Here's how the part is built. I have some questions about the finished solid (model axes, mm). A direction names the side the tool comes from. Coordinates: 2 decimals unless noted, no trailing zeros. Loops run counter-clockwise (first coordinate to the right, second up) from the corner with the lowest first, then second, coordinate; pieces in that order, holes last. Notation, with made-up numbers: M 52.5,42.5 L 66.5,42.5 A8 cw 66.5,53.5 Z; hole C 13.5,-8.75 d1. An arc over 180 degrees is marked long. Use one line per item in the form item = value. Start each with the question number.
(1) Imagine slicing it at C-C, the plane y = 15. Please give me the cut outline in (x, z).
(2) Imagine slicing it at A-A, the plane x = 0. Please give me the cut outline in (y, z) (3 decimals), and give its area (3 significant figures).
(3) Imagine slicing it at B-B, the plane z = 0. Please give me the cut outline in (x, y).
(4) On a 3-axis mill with a long thin cutter (end or side, diameter ignored), from which of +Z, -Z, +X, -X, +Y, -Y can I reach the whole of each face in a straight line? I mean faces 5 (the flat face through (-10.795, 6, -37)), 6 (the flat face through (26.87, 6.44, 27.98)), 7 (the cylindrical face through (-1.686, 5.106, -31.791)). Say none if no direction works.
(5) Imagine slicing it at D-D, the plane z = -16. Please give me the cut outline in (x, y), and give its area (3 significant figures).
(6) Thinking about a two-plate mould opening in Y: for faces 1 (the cylindrical face through (-0.237, 23.492, -37.256)), 2 (the flat face through (-37.7, 6.4, 9.3)), 3 (the cylindrical face through (25.737, 5.799, 19.004)), 4 (the cylindrical face through (-26.689, 5.106, 17.356)), which applies, +Y half, -Y half, draft (parallel to the pull), parting line (faces both ways), or undercut?
(7) Will these pins go through, and if not, where does the flat tip stop? P1, Ø12, axis at x = 32, z = -28, coming from the +Y side (1 decimal); P2, Ø2, axis at y = 45.5, z = -3, coming from the -X side; P3, Ø12, axis at y = 35.5, z = -22, coming from the +X side; P4, Ø5, axis at x = 9.5, z = -33.5, coming from the +Y side.
(8) Please list where these lines run through material, in increasing order: L1, parallel to X at y = 12.7, z = -37.5 (3 decimals); L2, parallel to X at y = 20.5, z = 2; L3, parallel to X at y = 7, z = 16.5.
```python
from build123d import *

# Parameters (mm, degrees)
SKETCH1_R               = 31.75
SKETCH1_R_2             = 20.32
BOSS_EXTRUDE1_DEPTH     = 50.8
BOSS_EXTRUDE2_START     = -12.7
SKETCH2_R               = 7.77875
BOSS_EXTRUDE2_DEPTH     = 14.591493
SKETCH2_2_R             = 7.77875
CUT_EXTRUDE1_DEPTH      = 12.977852
CIRPATTERN1_COUNT       = 3
F_1_4_CLEARANCE_HOLE1_D = 7.14248


with BuildPart() as part:
    # Sketch1 → Boss-Extrude1 (new body)
    with BuildSketch(Plane(origin=(0, 0, 0), x_dir=(1, 0, 0), z_dir=(0, 1, 0))):
        Circle(SKETCH1_R)
        Circle(SKETCH1_R_2, mode=Mode.SUBTRACT)
    extrude(amount=BOSS_EXTRUDE1_DEPTH)

    # Sketch2 → Boss-Extrude2 (add)
    with BuildSketch(Plane.XY.offset(-31.75).offset(BOSS_EXTRUDE2_START)):
        with BuildLine():
            Line((10.795, 12.7), (10.795, 0))
            Line((10.795, 0), (-10.795, 0))
            Line((-10.795, 0), (-10.795, 12.7))
            ThreePointArc((-10.795, 12.7), (0, 23.495), (10.795, 12.7))
        make_face()
        with Locations((0, 12.7)):
            Circle(SKETCH2_R, mode=Mode.SUBTRACT)
    boss_extrude2 = extrude(amount=BOSS_EXTRUDE2_DEPTH)

    # Sketch2<2> → Cut-Extrude1 (cut)
    with BuildSketch(Plane.XY.offset(-31.75)):
        with Locations((0, 12.7)):
            Circle(SKETCH2_2_R)
    cut_extrude1 = extrude(amount=CUT_EXTRUDE1_DEPTH, mode=Mode.SUBTRACT)

    # CirPattern1: Boss-Extrude2, Cut-Extrude1 ×3 about axis
    cirpattern1_axis = Axis((0, 0, 0), (0, 1, 0))
    for i in range(1, CIRPATTERN1_COUNT):
        add(boss_extrude2.rotate(cirpattern1_axis, i * 360 / CIRPATTERN1_COUNT))
        add(cut_extrude1.rotate(cirpattern1_axis, i * 360 / CIRPATTERN1_COUNT), mode=Mode.SUBTRACT)

    # 1/4 Clearance Hole1 (through all)
    with Locations(Plane(origin=(0, 50.8, 0), x_dir=(1, 0, 0), z_dir=(0, 1, 0))):
        with Locations((-25.4, 0), (25.4, 0)):
            Hole(F_1_4_CLEARANCE_HOLE1_D / 2)


solid = part.part
```
Answer:
q1.outline = M -43.77,13.09 L -31.21,5.84 A31.75 ccw -10.55,-29.95 L -10.55,-44.45 L -7.43,-44.45 L -7.43,-18.91 A20.32 cw -20.09,3.02 L -42.21,15.79 Z; M -34.78,28.66 L -12.66,15.89 A20.32 cw 12.66,15.89 L 34.78,28.66 L 33.22,31.36 L 20.66,24.11 A31.75 ccw -20.66,24.11 L -33.22,31.36 Z; M 7.43,-44.45 L 10.55,-44.45 L 10.55,-29.95 A31.75 ccw 31.21,5.84 L 43.77,13.09 L 42.21,15.79 L 20.09,3.02 A20.32 cw 7.43,-18.91 Z; hole C -25.4,0 d7.14; hole C 25.4,0 d7.14
q2.outline = M 0,-44.45 L 4.921,-44.45 L 4.921,-20.32 L 0,-20.32 Z; M 0,20.32 L 50.8,20.32 L 50.8,31.75 L 0,31.75 Z; M 20.479,-44.45 L 23.495,-44.45 L 23.495,-31.75 L 50.8,-31.75 L 50.8,-20.32 L 20.479,-20.32 Z
q2.area = 1,080 mm²
q3.outline = M -31.75,0 L -28.97,0 L -28.97,50.8 L -31.75,50.8 Z; M -21.83,0 L -20.32,0 L -20.32,50.8 L -21.83,50.8 Z; M 20.32,0 L 21.83,0 L 21.83,50.8 L 20.32,50.8 Z; M 28.97,0 L 31.75,0 L 31.75,50.8 L 28.97,50.8 Z
q4.face_5 = -Z, -X, +Y, -Y
q4.face_6 = +Z, +Y, -Y
q4.face_7 = -Z
q5.outline = M -27.42,0 L -12.53,0 L -12.53,50.8 L -27.42,50.8 Z; M 12.53,0 L 27.42,0 L 27.42,50.8 L 12.53,50.8 Z
q5.area = 1,510 mm²
q6.face_1 = +Y half
q6.face_2 = draft
q6.face_3 = undercut
q6.face_4 = undercut
q7.P1 = through
q7.P2 = -31.69
q7.P3 = 27.42
q7.P4 = 20.92
q8.L1 = -10.795 to -7.779, 7.779 to 10.795
q8.L2 = -31.69 to -28.36, -22.44 to -20.22, 20.22 to 22.44, 28.36 to 31.69
q8.L3 = -41.8 to -39.17, -17.99 to -11.86, 11.86 to 17.99, 39.17 to 41.8
